Source: three-view drawing plus pictorial views. Frame: mm from the lowest corner of the part. A direction names the side the tool comes from. Give positions to 0.01 mm unless a question says otherwise; leave off trailing zeros. Loops run counter-clockwise (first coordinate to the right, second up) from the corner with the lowest first, then second, coordinate; pieces in that order, holes last. Notation, with made-up numbers: M 81.5,-36.5 L 92.5,-36.5 A18 ccw 92.5,-4.5 Z; hole C -25.75,80 d5. An arc over 180 degrees is marked long. One line per item, written item: value. Start each with the question number.
(1) Ray query, line 1 along X through (y, z) = (140, 69.5); line 2 along Y through (x, z) = (66.5, 115.5). Return the intervals inside material, ascending. Write a range as from..to.
(2) Section C-C on z = 57.5. Output: boundary loops of the cut face in (x, y).
(3) Section A-A on x = 23. Output: boundary loops of the cut face in (y, z).
(4) Section D-D on z = 94.5. Output: boundary loops of the cut face in (x, y), plus the area to 3 significant figures.
(5) Section B-B on y = 39. Output: boundary loops of the cut face in (x, z), plus the area to 3 significant figures.
(6) Access query for the marked faces 1, 2 and 3. Directions: +Z, -Z, +X, -X, +Y, -Y. A direction counts if a zero-diameter tool reaches every point of the face in a straight line with its end or side. Return the directions, or none.
(7) Pin query (flat end, axial travel): P1, Ø10, axis at y = 116.5, z = 69, coming from the +X side. Return the tip coordinate at first contact, or that it passes through.
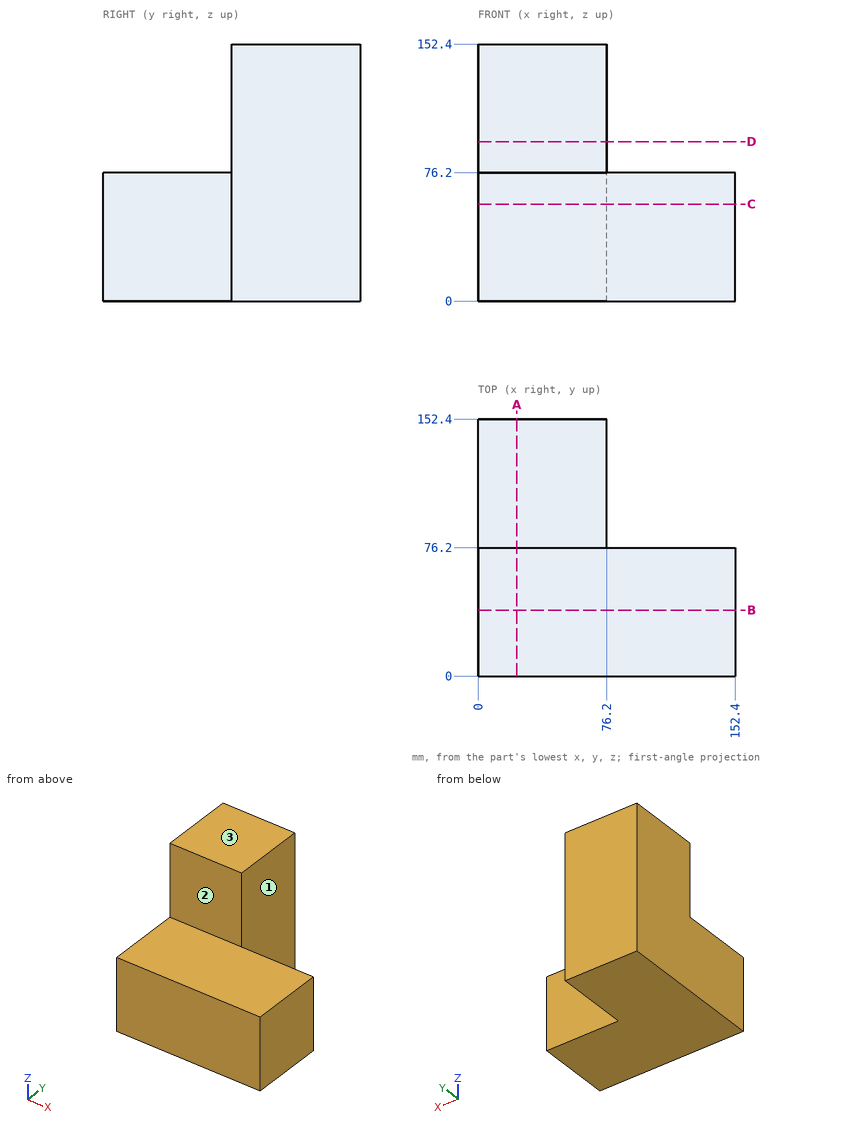
Output values:
1. line 1: x = 0..76.2
1. line 2: y = 76.2..152.4
2. outline: M 0,0 L 152.4,0 L 152.4,76.2 L 76.2,76.2 L 76.2,152.4 L 0,152.4 Z
3. outline: M 0,0 L 152.4,0 L 152.4,152.4 L 76.2,152.4 L 76.2,76.2 L 0,76.2 Z
4. outline: M 0,76.2 L 76.2,76.2 L 76.2,152.4 L 0,152.4 Z
4. area: 5,810 mm²
5. outline: M 0,0 L 152.4,0 L 152.4,76.2 L 0,76.2 Z
5. area: 11,600 mm²
6. face 1: +Z, -Z, +X, +Y
6. face 2: +Z, +X, -X, -Y
6. face 3: +Z, +X, -X, +Y, -Y
7. P1: stops at x = 76.2
